from build123d import *

# Parameters (mm, degrees)
SKETCH1_W           = 105
SKETCH1_H           = 5
SKETCH1_W_2         = 10
SKETCH1_H_2         = 50
BOSS_EXTRUDE1_DEPTH = 5
SKETCH2_R           = 1.75
CUT_EXTRUDE1_DEPTH  = 5
SKETCH3_R           = 1.75
CUT_EXTRUDE2_DEPTH  = 10


with BuildPart() as part:
    # Sketch1 → Boss-Extrude1 (new body)
    with BuildSketch(Plane.XY):
        Polygon((-35, 0), (0, 0), (0, 50), (-35, 50), (-140, 50), (-140, 0), align=None)
        Polygon((0, 50), (0, 0), (35, 0), (140, 0), (140, 50), (35, 50), align=None)
        with Locations((-87.5, -2.5)):
            Rectangle(SKETCH1_W, SKETCH1_H)
        with Locations((87.5, -2.5)):
            Rectangle(SKETCH1_W, SKETCH1_H)
        with Locations((-87.5, 52.5)):
            Rectangle(SKETCH1_W, SKETCH1_H)
        with Locations((87.5, 52.5)):
            Rectangle(SKETCH1_W, SKETCH1_H)
        with Locations((-145, 25)):
            Rectangle(SKETCH1_W_2, SKETCH1_H_2)
        with Locations((145, 25)):
            Rectangle(SKETCH1_W_2, SKETCH1_H_2)
    extrude(amount=BOSS_EXTRUDE1_DEPTH)

    # Sketch2 → Cut-Extrude1 (cut)
    with BuildSketch(Plane.XY.offset(5)):
        with Locations((-123.25, -2.5)):
            Circle(SKETCH2_R)
        with Locations(Location((-51.75, -2.5, 0), (0, 0, 180))):
            Circle(SKETCH2_R)
        with Locations((51.75, -2.5)):
            Circle(SKETCH2_R)
        with Locations(Location((123.25, -2.5, 0), (0, 0, 180))):
            Circle(SKETCH2_R)
        with Locations((123.25, 52.5)):
            Circle(SKETCH2_R)
        with Locations(Location((51.75, 52.5, 0), (0, 0, 180))):
            Circle(SKETCH2_R)
        with Locations((-51.75, 52.5)):
            Circle(SKETCH2_R)
        with Locations(Location((-123.25, 52.5, 0), (0, 0, 180))):
            Circle(SKETCH2_R)
    extrude(amount=-CUT_EXTRUDE1_DEPTH, mode=Mode.SUBTRACT)

    # Sketch3 → Cut-Extrude2 (cut)
    with BuildSketch(Plane.XY.offset(5)):
        with Locations((-145, 25)):
            Circle(SKETCH3_R)
        with Locations((145, 25)):
            Circle(SKETCH3_R)
    extrude(amount=-CUT_EXTRUDE2_DEPTH, mode=Mode.SUBTRACT)


solid = part.part
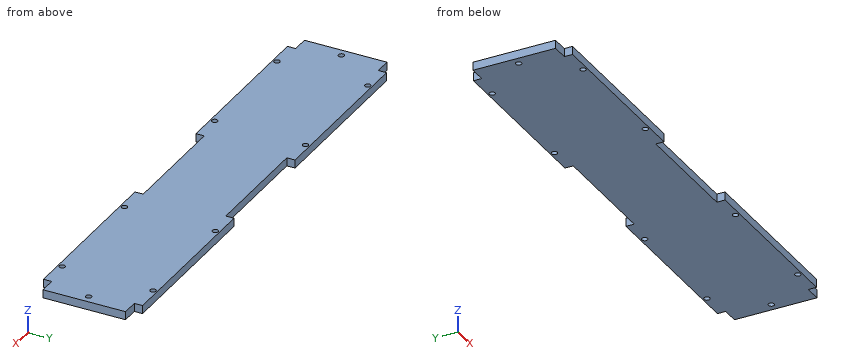
The listing builds one solid part. Answer for the finished solid, in the listing's coordinates (mm). Round coordinates to 2 decimals unless told otherwise and drop trailing zeros. Write each loop counter-clockwise with the first axis right and the second up, starting at its lowest first coordinate (ties: lowest second). Pieces come first, ordered by that corner, then holes. Notation, with made-up numbers: M 74,30 L 103,30 A30 ccw 103,67 Z; hole C 26.5,72 d8. An arc over 180 degrees is marked long. Write each question's results on one line, items separated by ' | '. Start each with the question number.
(1) Find the intervals of material crossed by line 1 (Y direction, x = -123.25, z = 1.85); line 2 (Y direction, x = -145, z = 3.85); line 3 (X direction, y = 51, z = 1.1), in increasing order.
(2) The part is cut by section B-B, the plane x = -3. Write down the section's boundary in (y, z).
(3) Each of these flat-tipped pins is pushed along its axis until it touches: P1, Ø2.5, axis at x = 144, z = 2.5, coming from the -Y side; P2, Ø2.5, axis at y = -2.5, z = 1.5, coming from the -X side; P3, Ø8, axis at x = 114.5, y = 43, coming from the -Z side; P4, Ø2.5, axis at y = -1.5, z = 1.5, coming from the +X side. Where does it stop, or does it pass through?
(4) The part is cut by section A-A, the plane z = 4.05. Give the number of separate pieces and of enclosed holes in the cut face, and give its area (3 significant figures).
Worked answers:
1) line 1: y = -5 to -4.25, -0.75 to 50.75, 54.25 to 55 | line 2: y = 0 to 23.25, 26.75 to 50 | line 3: x = -140 to -124.15, -122.35 to -52.65, -50.85 to -35, 35 to 50.85, 52.65 to 122.35, 124.15 to 140
2) outline: M 0,0 L 50,0 L 50,5 L 0,5 Z
3) P1: stops at y = 0 | P2: stops at x = -140 | P3: stops at z = 0 | P4: stops at x = 140
4) separate pieces: 1 | enclosed holes: 10 | area: 17,000 mm²
